Autodesk Inventor part; units mm, degrees
ref_plane "YZ Plane" through (0, 0, 0) normal (1, 0, 0) x (0, 1, 0)
ref_plane "XZ Plane" through (0, 0, 0) normal (0, 1, 0) x (-1, 0, 0)
ref_plane "XY Plane" through (0, 0, 0) normal (0, 0, 1) x (1, 0, 0)
sketch "Sketch1" plane through (0, 0, 0) normal (0, 0, 1) x (1, 0, 0)
  circle A0 centre (0, 0) radius 10
  arc A1 (-1.4142, 15.5) -> (1.4142, 15.5) centre (0, 15) ccw
  line L0 (1.4142, 15.5) -> (4.4142, 15.5)
  line L1 (-1.4142, 15.5) -> (-4.4142, 15.5)
  line L2 (-4.4142, 15.5) -> (-5.6974, 12.7883)
  line L3 (4.4142, 15.5) -> (5.6974, 12.7883)
  arc A2 (-12.7163, -8.9747) -> (-14.1305, -6.5253) centre (-12.9904, -7.5) ccw
  line L4 (-14.1305, -6.5253) -> (-15.6305, -3.9272)
  line L5 (-12.7163, -8.9747) -> (-11.2163, -11.5728)
  line L6 (-11.2163, -11.5728) -> (-8.2263, -11.3282)
  line L7 (-15.6305, -3.9272) -> (-13.9237, -1.4601)
  arc A3 (14.1305, -6.5253) -> (12.7163, -8.9747) centre (12.9904, -7.5) ccw
  line L8 (12.7163, -8.9747) -> (11.2163, -11.5728)
  line L9 (14.1305, -6.5253) -> (15.6305, -3.9272)
  line L10 (15.6305, -3.9272) -> (13.9237, -1.4601)
  line L11 (11.2163, -11.5728) -> (8.2263, -11.3282)
  arc A4 (-5.6974, 12.7883) -> (-13.9237, -1.4601) centre (0, 0) ccw
  arc A5 (-8.2263, -11.3282) -> (8.2263, -11.3282) centre (0, 0) ccw
  arc A6 (13.9237, -1.4601) -> (5.6974, 12.7883) centre (0, 0) ccw
  dimension "d0" = 20
  dimension "d1" = 3
  dimension "d3" = 15
  dimension "d4" = 3
  dimension "d5" = 0.5
  dimension "d6" = 3
  dimension "d9" = 360
  dimension "d11" = 14
extrude "Extrusion1" add sketch "Sketch1" along normal blind 4
chamfer "Chamfer1" distance 0.3 angle 45 2 edges at (-10, 0, 0) (-10, 0, 4)
properties part number "filament_guide_element" material "ABS Plastic"
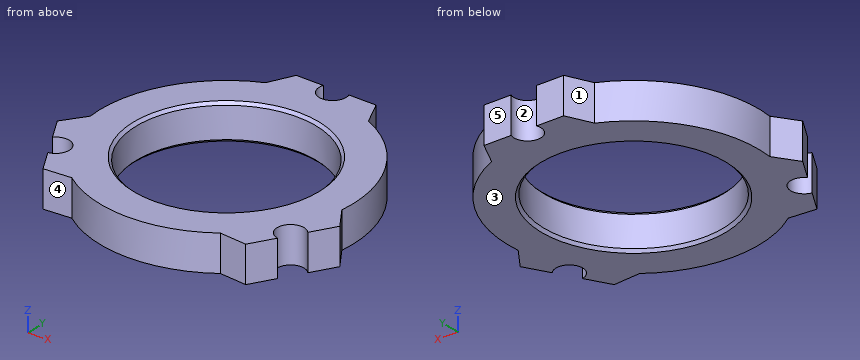
Design review of the part built by this model. Coordinates are the model's own, in mm. Face numbers are marked on the shaded views. A direction names the side the tool comes from. Give positions to 0.01 mm unless a question says otherwise; leave off trailing zeros. Loops run counter-clockwise (first coordinate to the right, second up) from the corner with the lowest first, then second, coordinate; pieces in that order, holes last. Notation, with made-up numbers: M 67.25,57.5 L 85.25,57.5 A31 ccw 85.25,92.5 Z; hole C 74.5,71.25 d9. An arc over 180 degrees is marked long. Answer as a JSON object with one key per item and string values.
Item 1: For P1, Ø2.5, axis at x = 12.99, y = -7.5, coming from the -Z side, flat-tipped, find the tip position at first contact; note if it passes through.
Output values:
{"P1": "passes through"}
Item 2: Machinability: for the marked faces 4 and 5, which of the approach directions +Z, -Z, +X, -X, +Y, -Y give a long, thin tool a straight path to every point of the face, cutting with its end or side? Answer none if there is none.
Output values:
{"face 4": "+Z, -Z, -Y", "face 5": "+Z, -Z, +X, -X, +Y"}
Item 3: Mouldability with a two-part tool opening along Y and no side actions: class the marked faces 1, 2 and 3 as pulls with the +Y half, pulls with the -Y half, needs draft (parallel to the pull), parting line crosses it, or undercut.
Output values:
{"face 1": "pulls with the +Y half", "face 2": "undercut", "face 3": "needs draft"}
Item 4: We need section B-B (x = 12). State the section outline as (y, z) points.
Output values:
{"outline": "M -10.22,0 L -8.63,0 L -8.63,4 L -10.22,4 Z; M -6.37,0 L 7.21,0 L 7.21,4 L -6.37,4 Z"}
Item 5: We need section A-A (y = 0). State the section outline as (x, z) points.
Output values:
{"outline": "M -14,0 L -10.3,0 L -10,0.3 L -10,3.7 L -10.3,4 L -14,4 Z; M 10,0.3 L 10.3,0 L 14,0 L 14,4 L 10.3,4 L 10,3.7 Z"}
Item 6: We need section C-C (z = 1.3). State the section outline as (x, y) points, and give its area (3 significant figures).
Output values:
{"outline": "M -15.63,-3.93 L -14.13,-6.53 A1.5 cw long -12.72,-8.97 L -11.22,-11.57 L -8.23,-11.33 A14 ccw 8.23,-11.33 L 11.22,-11.57 L 12.72,-8.97 A1.5 cw long 14.13,-6.53 L 15.63,-3.93 L 13.92,-1.46 A14 ccw 5.7,12.79 L 4.41,15.5 L 1.41,15.5 A1.5 cw long -1.41,15.5 L -4.41,15.5 L -5.7,12.79 A14 ccw -13.92,-1.46 Z; hole C 0,0 d20", "area": "341 mm2"}
Item 7: We need section D-D (y = 15). State the section outline as (x, z) points, and give its area (3 significant figures).
Output values:
{"outline": "M -4.65,0 L -1.5,0 L -1.5,4 L -4.65,4 Z; M 1.5,0 L 4.65,0 L 4.65,4 L 1.5,4 Z", "area": "25.2 mm2"}
Item 8: Wall thickness on line 1 along Y through (x, z) = (0, 2.5); line 2 along X through (y, z) = (-7.5, 0.95); line 3 along Y through (x, z) = (2, 3.4): over which ranges is each line inside the solid? List them lowest first.
Output values:
{"line 1": "y = -14 to -10, 10 to 13.5", "line 2": "x = -11.49 to -6.61, 6.61 to 11.49", "line 3": "y = -13.86 to -9.8, 9.8 to 15.5"}
